from build123d import *

# Parameters (mm, degrees)
SKETCH_1_R          = 2.75
EXTRUDE_1_DEPTH     = 1
SKETCH_2_R          = 1.5
EXTRUDE_2_DEPTH     = 8
SKETCH_3_W          = 1
SKETCH_3_H          = 1
CUT_EXTRUDE_1_DEPTH = 0.5


with BuildPart() as part:
    # ｽｹｯﾁ1 → ﾎﾞｽ - 押し出し1 (new body)
    with BuildSketch(Plane.XY):
        Circle(SKETCH_1_R)
    extrude(amount=EXTRUDE_1_DEPTH)

    # ｽｹｯﾁ2 → ﾎﾞｽ - 押し出し2 (add)
    with BuildSketch(Plane.XY.offset(1)):
        Circle(SKETCH_2_R)
    extrude(amount=EXTRUDE_2_DEPTH)

    # ｽｹｯﾁ3 → ｶｯﾄ - 押し出し1 (cut)
    with BuildSketch(Plane(origin=(0, 0, 0), x_dir=(-1, 0, 0), z_dir=(0, 0, -1))):
        with Locations((0, 1)):
            Rectangle(SKETCH_3_W, SKETCH_3_H)
        Rectangle(SKETCH_3_W, SKETCH_3_H)
        with Locations((1, 0)):
            Rectangle(SKETCH_3_W, SKETCH_3_H)
        with Locations((-1, 0)):
            Rectangle(SKETCH_3_W, SKETCH_3_H)
        with Locations((0, -1)):
            Rectangle(SKETCH_3_W, SKETCH_3_H)
    extrude(amount=-CUT_EXTRUDE_1_DEPTH, mode=Mode.SUBTRACT)


solid = part.part
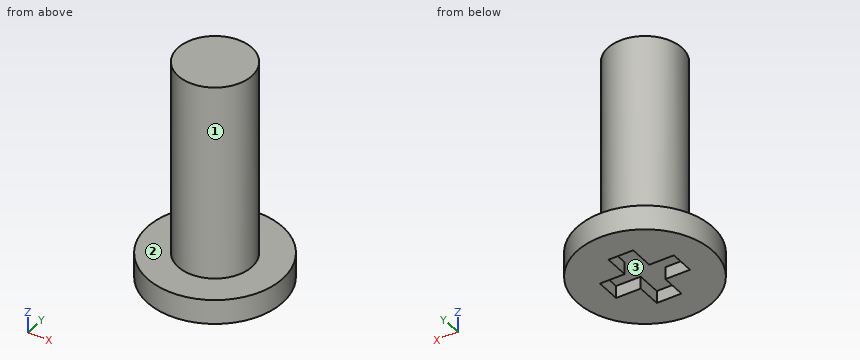
Model file for the job. Use its own axes, mm. Face numbers are marked on the shaded views. Give positions to 0.01 mm unless a question says otherwise; leave off trailing zeros. Loops run counter-clockwise (first coordinate to the right, second up) from the corner with the lowest first, then second, coordinate; pieces in that order, holes last.
1) Saw through at A-A (x = 0). Write the cut outline in (y, z).
2) Pull direction Y, two halves, no side cores. Call the marked faces 1, 2 and 3: +Y half, -Y half, draft (parallel to the pull), parting line (faces both ways), or undercut.
3) Wall check: line 1 (Z direction, x = -0.55, y = 2.45); line 2 (Z direction, x = 0.7, y = 0.15); line 3 (Y direction, x = 0.5, z = 5). Give the ranges that are in metal, low to high.
4) Flat gauge pins, fed straight in: pin 1 Ø0.6 at (x, z) = (-1, 0.5) entering from +Y; pin 2 Ø3 at (x, y) = (0.5, 1.5) entering from +Z; pin 3 Ø3 at (y, z) = (-1.5, 5.5) entering from +X; pin 4 Ø1 at (x, z) = (1, 5.5) entering from -Y. Where does each tip first touch, or does it go through?
5) Saw through at C-C (z = 2.5). Write the cut outline in (x, y).
6) Saw through at D-D (y = -2). Write the cut outline in (x, z).
Answer block:
1. outline: (-2.75, 0) - (-1.5, 0) - (-1.5, 0.5) - (1.5, 0.5) - (1.5, 0) - (2.75, 0) - (2.75, 1) - (1.5, 1) - (1.5, 9) - (-1.5, 9) - (-1.5, 1) - (-2.75, 1) - close
2. face 1: parting line
2. face 2: draft
2. face 3: undercut
3. line 1: z = 0 to 1
3. line 2: z = 0.5 to 9
3. line 3: y = -1.41 to 1.41
4. pin 1: stops at y = 2.66
4. pin 2: stops at z = 9
4. pin 3: stops at x = 1.5
4. pin 4: stops at y = -1.41
5. outline: circle Ø3 at (0, 0)
6. outline: (-1.89, 0) - (1.89, 0) - (1.89, 1) - (-1.89, 1) - close
